Could you check a few things on this model? Use its own coordinates, in mm. Face numbers are marked on the shaded views. Round coordinates to 2 decimals unless told otherwise and drop trailing zeros. Write each loop counter-clockwise with the first axis right and the second up, starting at its lowest first coordinate (ties: lowest second). Pieces come first, ordered by that corner, then holes. Notation, with made-up numbers: (31, 25) -> (38, 25) arc R14 cw to (38, 42) -> close; hole circle Ø9 at (-3.75, 17). An arc over 180 degrees is marked (long way). One line per question, with ' | ' between items. Start each with the question number.
1. Imagine slicing it at C-C, the plane y = 5.25. List the corners of the cut face in (x, z) for me.
2. Thinking about a two-plate mould opening in X: for the marked faces 1, 2 and 3, which applies, released by +X, released by -X, zero draft, split by the parting line, or undercut?
3. Imagine slicing it at D-D, the plane y = 2.75. List the corners of the cut face in (x, z) for me.
4. For pin 1 Ø1 at (y, z) = (4, 2.5) entering from -X; pin 2 Ø3 at (y, z) = (5, -3.5) entering from -X; pin 3 Ø1.5 at (x, y) = (9.5, 4) entering from -Z, each with a flat end and sliding along its axis, tell me the tip position at first contact or that it passes through.
5. If I drill on line 1 along X through (y, z) = (5.75, 0); line 2 along Y through (x, z) = (-14, 9.5); line 3 along X through (y, z) = (7.5, 0), over which ranges is the centre line in solid material (lowest first)? Write a range as [from, to].
6. Imagine slicing it at A-A, the plane z = 0. List the corners of the cut face in (x, y) for me.
7. Imagine slicing it at B-B, the plane x = 9.5. List the corners of the cut face in (y, z) for me.
from build123d import *

# Parameters (mm, degrees)
SKETCH_1_R          = 17.5
SKETCH_1_R_2        = 10
EXTRUDE_1_DEPTH     = 10
SKETCH_4_R          = 17.5
SKETCH_4_R_2        = 16
CUT_EXTRUDE_1_DEPTH = 1


with BuildPart() as part:
    # 草图1 → 凸台-拉伸1 (new body)
    with BuildSketch(Plane(origin=(0, 0, 0), x_dir=(1, 0, 0), z_dir=(0, 1, 0))):
        with Locations(Location((0, 0, 0), (0, 0, 270))):
            Circle(SKETCH_1_R)
        with Locations(Location((0, 0, 0), (0, 0, 270))):
            Circle(SKETCH_1_R_2, mode=Mode.SUBTRACT)
    extrude(amount=EXTRUDE_1_DEPTH)

    # 草图4 → 切除-拉伸1 (cut, symmetric)
    with BuildSketch(Plane(origin=(0, 5, 0), x_dir=(1, 0, 0), z_dir=(0, 1, 0))):
        with Locations(Location((0, 0, 0), (0, 0, 270))):
            Circle(SKETCH_4_R)
        with Locations(Location((0, 0, 0), (0, 0, 270))):
            Circle(SKETCH_4_R_2, mode=Mode.SUBTRACT)
    extrude(amount=CUT_EXTRUDE_1_DEPTH, both=True, mode=Mode.SUBTRACT)


solid = part.part
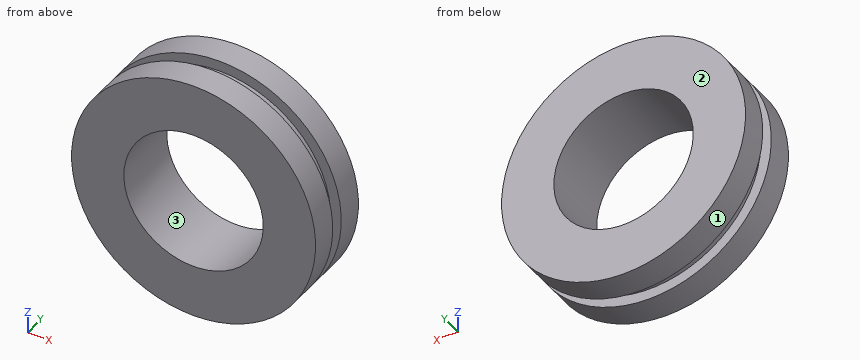
Geometry results:
1) outline: circle Ø32 at (0, 0); hole circle Ø20 at (0, 0)
2) face 1: split by the parting line | face 2: zero draft | face 3: undercut
3) outline: circle Ø35 at (0, 0); hole circle Ø20 at (0, 0)
4) pin 1: stops at x = -17.39 | pin 2: stops at x = -17.34 | pin 3: stops at z = -15.16
5) line 1: x = [-16, -10], [10, 16] | line 2: y = [0, 4], [6, 10] | line 3: x = [-17.5, -10], [10, 17.5]
6) outline: (-17.5, 0) -> (-10, 0) -> (-10, 10) -> (-17.5, 10) -> (-17.5, 6) -> (-16, 6) -> (-16, 4) -> (-17.5, 4) -> close; (10, 0) -> (17.5, 0) -> (17.5, 4) -> (16, 4) -> (16, 6) -> (17.5, 6) -> (17.5, 10) -> (10, 10) -> close
7) outline: (0, -14.7) -> (4, -14.7) -> (4, -12.87) -> (6, -12.87) -> (6, -14.7) -> (10, -14.7) -> (10, -3.12) -> (0, -3.12) -> close; (0, 3.12) -> (10, 3.12) -> (10, 14.7) -> (6, 14.7) -> (6, 12.87) -> (4, 12.87) -> (4, 14.7) -> (0, 14.7) -> close
